Input: part model. Units: mm. Frame: model coordinates. A direction names the side the tool comes from. Coordinates: 2 decimals unless noted, no trailing zeros. Order: outer loops, then holes, each group sorted by start corner. A loop starts at its lowest first (then second) coordinate and runs counter-clockwise, first axis right, second up. Notation, with made-up numbers: (-8, 15.25) - (44, 15.25) arc R34 ccw to (44, 50.25) - close; hole circle Ø1 at (41.25, 85). An arc over 180 degrees is marked (long way). Answer as CSV lines item,"result". Start each with the question number.
Item 1: Material intervals for line 1 along Y through (x, z) = (0, 19); line 2 along Z through (x, y) = (-0.25, 4.5); line 3 along Y through (x, z) = (-1.25, 31), sorted ascending.
Item 2: Access query for faces 1 (the flat face through (-1.5, 4, 38)), 2 (the flat face through (2, 6, 5)), 3 (the flat face through (-2, 6, 5)). Directions: +Z, -Z, +X, -X, +Y, -Y. A direction counts if a zero-diameter tool reaches every point of the face in a straight line with its end or side. Return the directions, or none.
Item 3: Section A-A (x = 0). Output: boundary loops of the cut face in (y, z), and give its area (3 significant figures).
Item 4: Section C-C (y = 5.5). Output: boundary loops of the cut face in (x, z), and give its area (3 significant figures).
Item 5: Draft query along X for faces 4 (the conical face through (-0.184, -4.632, 39.865)), 5 (the flat face through (0, 7, 5)), 6 (the flat face through (1.5, 4, 37)). Return one class per face: +X half, -X half, draft (parallel to the pull), parting line (faces both ways), or undercut.
Item 6: Section B-B (z = 15). Output: boundary loops of the cut face in (x, y), and give its area (3 significant figures).
Item 7: First-contact query: pin 1 (2 mm diameter, centred on x = 3, z = 18.5, fed in from +Y); pin 2 (1.9 mm diameter, centred on y = 6, z = 5, fed in from -X); pin 3 (0.9 mm diameter, centred on x = -0.5, z = 36.5, fed in from +Y). Flat tips, straight axial feed; report the tip coordinate or a pass-through.
from build123d import *

# Parameters (mm, degrees)
BOSS_EXTRUDE1_DEPTH = 10
SKETCH2_R           = 5
BOSS_EXTRUDE2_DEPTH = 30
CUT_EXTRUDE1_START  = 3
CUT_EXTRUDE1_DEPTH  = 38.914545091
CHAMFER1_SIZE       = 0.5


with BuildPart() as part:
    # Sketch1 → Boss-Extrude1 (new body)
    with BuildSketch(Plane.XY):
        with BuildLine():
            Line((-2, 7), (2, 7))
            Line((2, 7), (2, 4.582575695))
            ThreePointArc((2, 4.582575695), (0, -5), (-2, 4.582575695))
            Line((-2, 4.582575695), (-2, 7))
        make_face()
    extrude(amount=BOSS_EXTRUDE1_DEPTH)

    # Sketch2 → Boss-Extrude2 (add)
    with BuildSketch(Plane.XY.offset(10)):
        with Locations(Location((0, 0, 0), (0, 0, 113.578178478))):
            Circle(SKETCH2_R)
    extrude(amount=BOSS_EXTRUDE2_DEPTH)

    # Sketch3 → Cut-Extrude1 (cut, through all)
    with BuildSketch(Plane(origin=(0, 0, 0), x_dir=(1, 0, 0), z_dir=(0, 1, 0)).offset(CUT_EXTRUDE1_START)):
        with BuildLine():
            Line((-1.5, -40), (-1.5, -35))
            ThreePointArc((-1.5, -35), (0, -33.5), (1.5, -35))
            Line((1.5, -35), (1.5, -40))
            ThreePointArc((1.5, -40), (0, -41.5), (-1.5, -40))
        make_face()
    extrude(amount=CUT_EXTRUDE1_DEPTH, mode=Mode.SUBTRACT)

    # Chamfer1
    chamfer1_edges = [part.edges().sort_by_distance(p)[0] for p in [
        (0.266933518, -4.992869565, 40),
    ]]
    chamfer(chamfer1_edges, length=CHAMFER1_SIZE)


solid = part.part
Determined:
1,line 1,"y = -5 to 5"
1,line 2,"z = 0 to 33.52"
1,line 3,"y = -4.84 to 4.84"
2,face 1,"+Z, +Y"
2,face 2,"+Z, -Z, +X, +Y"
2,face 3,"+Z, -Z, -X, +Y"
3,outline,"(-5, 0) - (7, 0) - (7, 10) - (5, 10) - (5, 33.5) - (3, 33.5) - (3, 40) - (-4.5, 40) - (-5, 39.5) - close"
3,area,"407 mm^2"
4,outline,"(-2, 0) - (2, 0) - (2, 10) - (-2, 10) - close"
4,area,"40.0 mm^2"
5,face 4,"parting line"
5,face 5,"draft"
5,face 6,"undercut"
6,outline,"circle Ø10 at (0, 0)"
6,area,"78.5 mm^2"
7,pin 1,"stops at y = 4.58"
7,pin 2,"stops at x = -2"
7,pin 3,"stops at y = 3"
